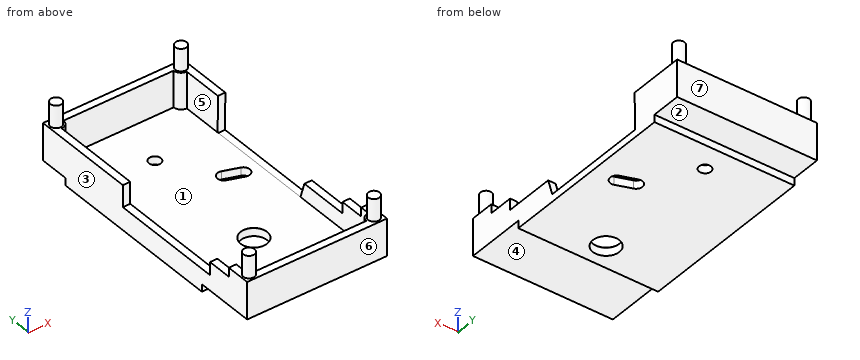
from build123d import *

# Parameters (mm, degrees)
SKETCH2_W                  = 23.9522
SKETCH2_H                  = 45.7962
SKETCH2_R                  = 2.2606
SKETCH2_R_2                = 1.016
BOSS_EXTRUDE1_DEPTH        = 6.35
SKETCH4_W                  = 21.4122
SKETCH4_H                  = 43.2562
CUT_EXTRUDE1_DEPTH         = 6.223
CUT_EXTRUDE3_DEPTH         = 2.54
CUT_EXTRUDE5_DEPTH         = 1.27
BOSS_EXTRUDE3_DEPTH        = 6.223
SKETCH12_R                 = 0.9652
BOSS_EXTRUDE13_DEPTH       = 3.81
BOSS_EXTRUDE15_OUTLINE_W   = 23.9522
BOSS_EXTRUDE15_OUTLINE_H   = 30.5562
BOSS_EXTRUDE15_OUTLINE_R   = 2.2606
BOSS_EXTRUDE15_OUTLINE_R_2 = 1.016
BOSS_EXTRUDE15_DEPTH       = 1.27


# Read off the part's stored shape, not the designer's step: Boss-Extrude15
with BuildPart() as part:
    # Sketch2 → Boss-Extrude1 (new body)
    with BuildSketch(Plane.XY):
        Rectangle(SKETCH2_W, SKETCH2_H)
        with Locations((0, -8.7249)):
            Circle(SKETCH2_R, mode=Mode.SUBTRACT)
        with Locations((0, 13.4747)):
            Circle(SKETCH2_R_2, mode=Mode.SUBTRACT)
        with BuildLine():
            Line((8.361518313, 5.139100055), (5.725634689, 6.065681687))
            ThreePointArc((5.725634689, 6.065681687), (4.333034634, 5.3975), (5.001216321, 4.004899945))
            Line((5.001216321, 4.004899945), (7.637099945, 3.078318313))
            ThreePointArc((7.637099945, 3.078318313), (9.0297, 3.7465), (8.361518313, 5.139100055))
        make_face(mode=Mode.SUBTRACT)
    extrude(amount=BOSS_EXTRUDE1_DEPTH)

    # Sketch4 → Cut-Extrude1 (cut)
    with BuildSketch(Plane.XY.offset(6.35)):
        Rectangle(SKETCH4_W, SKETCH4_H)
    extrude(amount=-CUT_EXTRUDE1_DEPTH, mode=Mode.SUBTRACT)

    # Sketch6 → Cut-Extrude3 (cut)
    with BuildSketch(Plane.ZY.offset(11.9761)):
        Polygon((4.826, -14.5669), (2.6162, -14.5669), (2.6162, 4.9911), (6.35, 4.9911), (6.35, -18.7833), (4.826, -18.7833), align=None)
    extrude(amount=-CUT_EXTRUDE3_DEPTH, mode=Mode.SUBTRACT)

    # Sketch8 → Cut-Extrude5 (cut)
    with BuildSketch(Plane(origin=(11.9761, 0, 0), x_dir=(0, 0, -1), z_dir=(1, 0, 0))):
        Polygon((-6.35, -18.7833), (-4.826, -18.7833), (-4.826, -14.5669), (-2.8956, -14.5669), (-2.8956, -6.0325), (0, -5.1181), (0, 13.4239), (-6.35, 13.3731), align=None)
    extrude(amount=-CUT_EXTRUDE5_DEPTH, mode=Mode.SUBTRACT)

    # Sketch10 → Boss-Extrude3 (add)
    with BuildSketch(Plane.XY.offset(0.127)):
        with BuildLine():
            ThreePointArc((-10.7061, 20.3581), (-9.808074388, 20.730074388), (-9.4361, 21.6281))
            Line((-9.4361, 21.6281), (-10.7061, 21.6281))
            Line((-10.7061, 21.6281), (-10.7061, 20.3581))
        make_face()
        with BuildLine():
            ThreePointArc((9.4361, 21.6281), (9.808074388, 20.730074388), (10.7061, 20.3581))
            Line((10.7061, 20.3581), (10.7061, 21.6281))
            Line((10.7061, 21.6281), (9.4361, 21.6281))
        make_face()
        with BuildLine():
            ThreePointArc((-9.4361, -21.6281), (-9.808074388, -20.730074388), (-10.7061, -20.3581))
            Line((-10.7061, -20.3581), (-10.7061, -21.6281))
            Line((-10.7061, -21.6281), (-9.4361, -21.6281))
        make_face()
        with BuildLine():
            Line((10.7061, -21.6281), (10.7061, -20.3581))
            ThreePointArc((10.7061, -20.3581), (9.808074388, -20.730074388), (9.4361, -21.6281))
            Line((9.4361, -21.6281), (10.7061, -21.6281))
        make_face()
    extrude(amount=BOSS_EXTRUDE3_DEPTH)

    # Sketch12 → Boss-Extrude13 (add)
    with BuildSketch(Plane.XY.offset(6.35)):
        with Locations(Location((-10.7061, 21.6281, 0), (0, 0, 180))):
            Circle(SKETCH12_R)
        with Locations(Location((10.7061, 21.6281, 0), (0, 0, 180))):
            Circle(SKETCH12_R)
        with Locations(Location((10.7061, -21.6281, 0), (0, 0, 180))):
            Circle(SKETCH12_R)
        with Locations(Location((-10.7061, -21.6281, 0), (0, 0, 180))):
            Circle(SKETCH12_R)
    extrude(amount=BOSS_EXTRUDE13_DEPTH)

    # Boss-Extrude15 outline → Boss-Extrude15 (add)
    with BuildSketch(Plane(origin=(0, 0, 0), x_dir=(-1, 0, 0), z_dir=(0, 0, -1))):
        with Locations((0, 2.54)):
            Rectangle(BOSS_EXTRUDE15_OUTLINE_W, BOSS_EXTRUDE15_OUTLINE_H)
        with Locations((0, -8.7249)):
            Circle(BOSS_EXTRUDE15_OUTLINE_R, mode=Mode.SUBTRACT)
        with BuildLine():
            ThreePointArc((-7.637099945, 3.078318313), (-9.0297, 3.7465), (-8.361518313, 5.139100055))
            Line((-8.361518313, 5.139100055), (-5.725634689, 6.065681687))
            ThreePointArc((-5.725634689, 6.065681687), (-4.333034634, 5.3975), (-5.001216321, 4.004899945))
            Line((-5.001216321, 4.004899945), (-7.637099945, 3.078318313))
        make_face(mode=Mode.SUBTRACT)
        with Locations((0, 13.4747)):
            Circle(BOSS_EXTRUDE15_OUTLINE_R_2, mode=Mode.SUBTRACT)
    extrude(amount=BOSS_EXTRUDE15_DEPTH)


solid = part.part
CAD build for the part. Positions are in the model's coordinates, mm. Face numbers are marked on the shaded views. A direction names the side the tool comes from. Coordinates: 2 decimals unless noted, no trailing zeros. Order: outer loops, then holes, each group sorted by start corner. A loop starts at its lowest first (then second) coordinate and runs counter-clockwise, first axis right, second up. Notation, with made-up numbers: (87, -37) -> (116, -37) arc R23 cw to (116, -24) -> close; hole circle Ø4 at (42, 12). An arc over 180 degrees is marked (long way). Answer in a Markdown table with one row per item.
1) Band-saw the part on D-D (x = -6.75). List the corners of the cut face in (y, z), and give its area (3 significant figures).
Check values:
| item | result |
|---|---|
| outline | (-22.9, 0) -> (-12.74, 0) -> (-12.74, -1.27) -> (17.82, -1.27) -> (17.82, 0) -> (22.9, 0) -> (22.9, 6.35) -> (21.63, 6.35) -> (21.63, 0.13) -> (-21.63, 0.13) -> (-21.63, 6.35) -> (-22.9, 6.35) -> close |
| area | 60.4 mm2 |
2) Drill centre lines: line 1 (Y direction, x = 0, z = -0.25); line 2 (X direction, y = 18, z = 6); line 3 (Y direction, x = 0.5, z = 3). Where is each one in solid material? Low to high.
Check values:
| item | result |
|---|---|
| line 1 | -12.74 to -10.99, -6.46 to 12.46, 14.49 to 17.82 |
| line 2 | -11.98 to -10.71, 10.71 to 11.98 |
| line 3 | -22.9 to -21.63, 21.63 to 22.9 |
3) Which spindle directions (+Z, -Z, +X, -X, +Y, -Y) get a long thin tool onto all of the face, cutting with end or side? Do the marked faces 1, 2 and 3. Say none if no direction does.
Check values:
| item | result |
|---|---|
| face 1 | +Z |
| face 2 | -Z, +X, -X, +Y |
| face 3 | +Z, -Z, -X, +Y, -Y |
4) Band-saw the part on B-B (y = -2). List the corners of the cut face in (x, z).
Check values:
| item | result |
|---|---|
| outline | (-11.98, -1.27) -> (11.98, -1.27) -> (11.98, 0) -> (10.71, 0) -> (10.71, 0.13) -> (-10.71, 0.13) -> (-10.71, 2.62) -> (-11.98, 2.62) -> close |
5) Flat gauge pins, fed straight in: P1, Ø6, axis at x = -4.5, y = 12.5, coming from the +Z side; P2, Ø1, axis at x = 11.5, y = -12, coming from the +Z side; P3, Ø1, axis at x = -11.5, y = -17.5, coming from the +Z side; P4, Ø2.5, axis at x = 0, y = -8.72, coming from the -Z side. Where does each tip first touch, or does it go through?
Check values:
| item | result |
|---|---|
| P1 | z = 0.13 |
| P2 | z = 2.9 |
| P3 | z = 4.83 |
| P4 | through |
6) Band-saw the part on C-C (z = 4). List the corners of the cut face in (x, y).
Check values:
| item | result |
|---|---|
| outline | (-11.98, -22.9) -> (11.98, -22.9) -> (11.98, -14.57) -> (10.71, -14.57) -> (10.71, -20.36) arc R1.27 ccw to (9.44, -21.63) -> (-9.44, -21.63) arc R1.27 ccw to (-10.71, -20.36) -> (-10.71, -14.57) -> (-11.98, -14.57) -> close; (-11.98, 4.99) -> (-10.71, 4.99) -> (-10.71, 20.36) arc R1.27 ccw to (-9.44, 21.63) -> (9.44, 21.63) arc R1.27 ccw to (10.71, 20.36) -> (10.71, 13.39) -> (11.98, 13.39) -> (11.98, 22.9) -> (-11.98, 22.9) -> close |
7) Band-saw the part on A-A (x = 0). List the corners of the cut face in (y, z), and give its area (3 significant figures).
Check values:
| item | result |
|---|---|
| outline | (-22.9, 0) -> (-12.74, 0) -> (-12.74, -1.27) -> (-10.99, -1.27) -> (-10.99, 0.13) -> (-21.63, 0.13) -> (-21.63, 6.35) -> (-22.9, 6.35) -> close; (-6.46, -1.27) -> (12.46, -1.27) -> (12.46, 0.13) -> (-6.46, 0.13) -> close; (14.49, -1.27) -> (17.82, -1.27) -> (17.82, 0) -> (22.9, 0) -> (22.9, 6.35) -> (21.63, 6.35) -> (21.63, 0.13) -> (14.49, 0.13) -> close |
| area | 51.3 mm2 |
8) Mould opens along Y. For the marked faces 4, 5, 6 and 7 say: pulls with the +Y half, pulls with the -Y half, needs draft (parallel to the pull), parting line crosses it, or undercut.
Check values:
| item | result |
|---|---|
| face 4 | needs draft |
| face 5 | undercut |
| face 6 | pulls with the -Y half |
| face 7 | pulls with the +Y half |
